Build history of the part. All positions in model axes, mm. Face numbers are marked on the shaded views. A direction names the side the tool comes from. Coordinates: 2 decimals unless noted, no trailing zeros. Loops run counter-clockwise (first coordinate to the right, second up) from the corner with the lowest first, then second, coordinate; pieces in that order, holes last.
(1) Flat gauge pins, fed straight in: P1, Ø0.8, axis at x = 1, z = -0.5, coming from the -Y side; P2, Ø0.8, axis at x = 0, y = -1.5, coming from the -Z side; P3, Ø8, axis at y = 12, z = 9.5, coming from the -X side; P4, Ø6, axis at y = 1.5, z = 12.5, coming from the +X side. Where does each tip first touch, or does it go through?
(2) Slice it at C-C (y = 4.5). Give the cut face in (x, z).
(3) Two-plate mould, pull along Y, no slides. Class the marked faces 3 and 4: pulls with the +Y half, pulls with the -Y half, needs draft (parallel to the pull), parting line crosses it, or undercut.
(4) Slice it at D-D (z = 8.5). Give the cut face in (x, y), and give its area (3 significant figures).
(5) Slice it at B-B (z = 4). Give the cut face in (x, y), and give its area (3 significant figures).
(6) Tool access for the marked faces 1 and 2: list every direction of +Z, -Z, +X, -X, +Y, -Y with a clear straight run to the whole face (end or side of a thin tool).
(7) Slice it at A-A (x = 0). Give the cut face in (y, z).
(8) Wall check: L1, parallel to Z at x = 1, y = -1; L2, parallel to Z at x = -1.6, y = 3; L3, parallel to Y at x = -0.1, z = 12. Give the ranges that are in metal, low to high.
Autodesk Inventor part; units mm, degrees
ref_plane "YZ Plane" through (0, 0, 0) normal (1, 0, 0) x (0, 1, 0)
ref_plane "XZ Plane" through (0, 0, 0) normal (0, 1, 0) x (-1, 0, 0)
ref_plane "XY Plane" through (0, 0, 0) normal (0, 0, 1) x (1, 0, 0)
sketch "Sketch1" plane through (0, 0, 0) normal (0, 0, 1) x (1, 0, 0)
  circle A0 centre (0, 0) radius 2.5
  dimension "d0" = 5
extrude "Extrusion1" add sketch "Sketch1" along normal blind 15
sketch "Sketch2" plane through (0, 0, 0) normal (0, 0, -1) x (-1, 0, 0)
  circle A0 centre (0, 0) radius 2.5
  line L0 (2.5, 0) -> (-2.5, 0)
  line L1 (-2.5, 0) -> (-2.5, 15)
  line L2 (-2.5, 15) -> (2.5, 15)
  line L3 (2.5, 15) -> (2.5, 0)
  dimension "d3" = 15
extrude "Extrusion2" add sketch "Sketch2" along normal blind 1 contours L0 A0 | A0 L1 L2 L3 picked at (0.6238, 0.5526)
sketch "Sketch3" plane through (0, 0, 0) normal (0, 0, 1) x (1, 0, 0)
  circle A0 centre (0, 4.5) radius 0.5
  point P0 (0, 0)
  dimension "d7" = 1
extrude "Extrusion3" add sketch "Sketch3" along normal blind 7
properties part number "pathFollower" material "Stainless Steel"
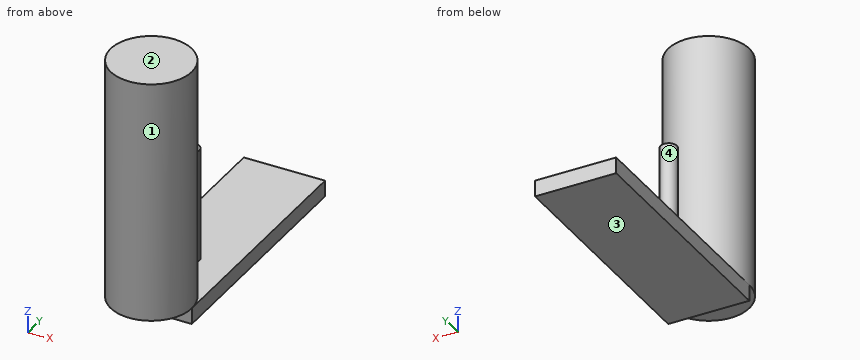
Response values:
1. P1: stops at y = 0
1. P2: stops at z = 0
1. P3: passes through
1. P4: stops at x = 2.5
2. outline: (-2.5, -1) - (2.5, -1) - (2.5, 0) - (0.5, 0) - (0.5, 7) - (-0.5, 7) - (-0.5, 0) - (-2.5, 0) - close
3. face 3: needs draft
3. face 4: undercut
4. outline: circle Ø5 at (0, 0)
4. area: 19.6 mm2
5. outline: circle Ø5 at (0, 0); circle Ø1 at (0, 4.5)
5. area: 20.4 mm2
6. face 1: +Z
6. face 2: +Z, +X, -X, +Y, -Y
7. outline: (-2.5, 0) - (0, 0) - (0, -1) - (15, -1) - (15, 0) - (5, 0) - (5, 7) - (4, 7) - (4, 0) - (2.5, 0) - (2.5, 15) - (-2.5, 15) - close
8. L1: z = 0 to 15
8. L2: z = -1 to 0
8. L3: y = -2.5 to 2.5
